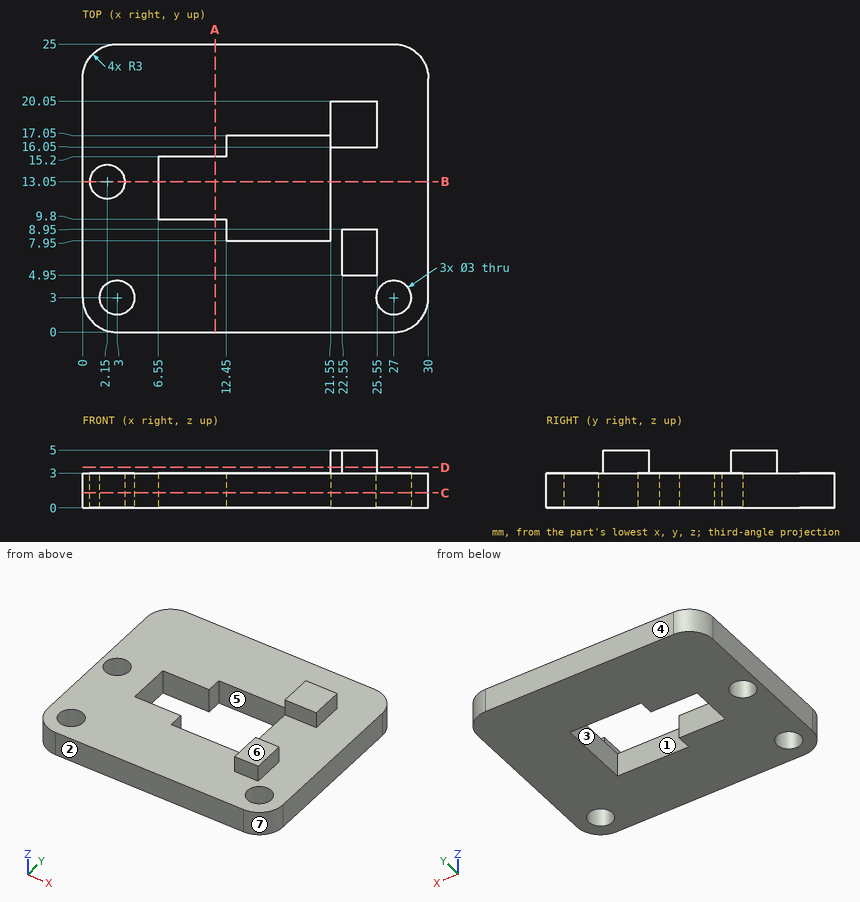
Print and shaded views of the part. All mm, measured from the part's lowest x, y and z. A direction names the side the tool comes from. Coordinates: 2 decimals unless noted, no trailing zeros. Write each loop counter-clockwise with the first axis right and the second up, starting at its lowest first coordinate (ties: lowest second). Pieces come first, ordered by that corner, then holes. Notation, with made-up numbers: (47, 43.5) - (59, 43.5) arc R22 cw to (59, 76.5) - close; hole circle Ø11 at (16.5, 4). An arc over 180 degrees is marked (long way). One line per question, with ' | ' between items. Start each with the question number.
Q1. Pin check, flat tips, straight feed: pin 1 (8 mm diameter, centred on x = 5.5, y = 6.5, fed in from +Z); pin 2 (1.6 mm diameter, centred on x = 23.5, z = 4, fed in from +Y); pin 3 (1 mm diameter, centred on x = 23, z = 4, fed in from -Y). Stop position of each tip, or through.
Q2. Cut at D-D, the plane z = 3.5. List the corners of the cut face in (x, y), then the cut area to 3 significant figures.
Q3. Pull direction Y, two halves, no side cores. Call the marked faces 4, 5, 6 and 7: pulls with the +Y half, pulls with the -Y half, needs draft (parallel to the pull), parting line crosses it, or undercut.
Q4. 3-axis set-ups, long thin cutter, end or side, ignore diameter. For the marked faces 1, 2 and 3: which of +Z, -Z, +X, -X, +Y, -Y reach the whole face in a straight line?
Q5. Cut at B-B, the plane y = 13.05. List the corners of the cut face in (x, z).
Q6. Drill centre lines: line 1 (Y direction, x = 2, z = 2.9); line 2 (X direction, y = 12.25, z = 2.3); line 3 (Y direction, x = 27, z = 1.4). Where is each one in solid material? Low to high. Write a range as [from, to].
Q7. Cut at A-A, the plane x = 11.5. List the corners of the cut face in (y, z).
Q8. Cut at C-C, the plane z = 1.3. List the corners of the cut face in (x, y), then the cut area to 3 significant figures.
Answer below:
1) pin 1: z = 3 | pin 2: y = 20.05 | pin 3: y = 4.95
2) outline: (21.55, 16.05) - (25.55, 16.05) - (25.55, 20.05) - (21.55, 20.05) - close; (22.55, 4.95) - (25.55, 4.95) - (25.55, 8.95) - (22.55, 8.95) - close | area: 28.0 mm^2
3) face 4: pulls with the +Y half | face 5: undercut | face 6: needs draft | face 7: pulls with the -Y half
4) face 1: +Z, -Z | face 2: +Z, -Z, +X, -X, -Y | face 3: +Z
5) outline: (0, 0) - (0.65, 0) - (0.65, 3) - (0, 3) - close; (3.65, 0) - (6.55, 0) - (6.55, 3) - (3.65, 3) - close; (21.55, 0) - (30, 0) - (30, 3) - (21.55, 3) - close
6) line 1: [0.17, 1.88], [4.12, 11.56], [14.54, 24.83] | line 2: [0, 0.88], [3.42, 6.55], [21.55, 30] | line 3: [0, 1.5], [4.5, 25]
7) outline: (0, 0) - (9.8, 0) - (9.8, 3) - (0, 3) - close; (15.2, 0) - (25, 0) - (25, 3) - (15.2, 3) - close
8) outline: (0, 3) arc R3 ccw to (3, 0) - (27, 0) arc R3 ccw to (30, 3) - (30, 22) arc R3 ccw to (27, 25) - (3, 25) arc R3 ccw to (0, 22) - close; hole circle Ø3 at (2.15, 13.05); hole circle Ø3 at (3, 3); hole (6.55, 9.8) - (12.45, 9.8) - (12.45, 7.95) - (21.55, 7.95) - (21.55, 17.05) - (12.45, 17.05) - (12.45, 15.2) - (6.55, 15.2) - close; hole circle Ø3 at (27, 3) | area: 606 mm^2
